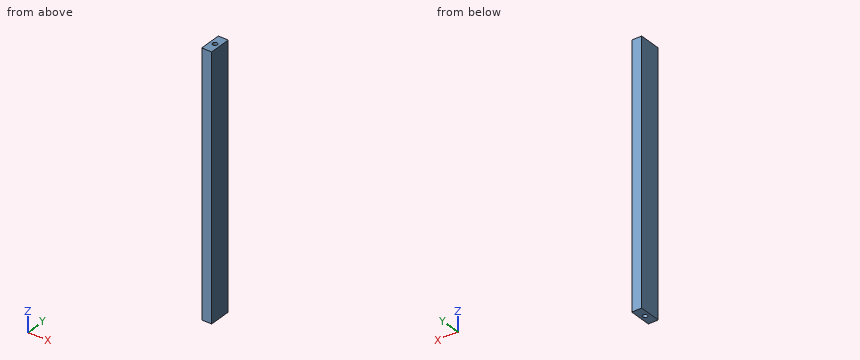
from build123d import *

# Parameters (mm, degrees)
SKETCH1_W           = 9
SKETCH1_H           = 20
BOSS_EXTRUDE1_DEPTH = 117.5
SKETCH2_R           = 2.1
CUT_EXTRUDE1_DEPTH  = 11


with BuildPart() as part:
    # Sketch1 → Boss-Extrude1 (new body, symmetric)
    with BuildSketch(Plane.XY):
        Rectangle(SKETCH1_W, SKETCH1_H)
    extrude(amount=BOSS_EXTRUDE1_DEPTH, both=True)

    # Sketch2 → Cut-Extrude1 (cut)
    with BuildSketch(Plane.XY.offset(117.5)):
        Circle(SKETCH2_R)
    cut_extrude1 = extrude(amount=-CUT_EXTRUDE1_DEPTH, mode=Mode.SUBTRACT)

    # Mirror1: Cut-Extrude1 across plane
    add(cut_extrude1.mirror(Plane.XY), mode=Mode.SUBTRACT)


solid = part.part
The listing builds one solid part. Answer for the finished solid, in the listing's coordinates (mm). Give positions to 0.01 mm unless a question says otherwise; leave off trailing zeros. Write each loop counter-clockwise with the first axis right and the second up, starting at its lowest first coordinate (ties: lowest second). Pieces come first, ordered by that corner, then holes.
Item 1: Section A-A, the plane y = 0 is taken. Write down the section's boundary in (x, z), plus the area to 3 significant figures.
Item 2: Flat-ended cylindrical pins translate along their axes: P1, Ø1.3, axis at x = -0.5, y = 0, coming from the -Z side; P2, Ø4.5, axis at x = 0, y = 0, coming from the +Z side. Find the tip coordinate at first contact, or state that the pin passes through.
Item 3: Find the intervals of material crossed by line 1 along Y through (x, z) = (0, -114.75); line 2 along Z through (x, y) = (0.25, -2), in increasing order.
Item 4: Section B-B, the plane x = 0 is taken. Write down the section's boundary in (y, z).
Completed:
1. outline: (-4.5, -117.5) - (-2.1, -117.5) - (-2.1, -106.5) - (2.1, -106.5) - (2.1, -117.5) - (4.5, -117.5) - (4.5, 117.5) - (2.1, 117.5) - (2.1, 106.5) - (-2.1, 106.5) - (-2.1, 117.5) - (-4.5, 117.5) - close
1. area: 2,020 mm2
2. P1: stops at z = -106.5
2. P2: stops at z = 117.5
3. line 1: y = -10 to -2.1, 2.1 to 10
3. line 2: z = -106.5 to 106.5
4. outline: (-10, -117.5) - (-2.1, -117.5) - (-2.1, -106.5) - (2.1, -106.5) - (2.1, -117.5) - (10, -117.5) - (10, 117.5) - (2.1, 117.5) - (2.1, 106.5) - (-2.1, 106.5) - (-2.1, 117.5) - (-10, 117.5) - close
